Verification items for the finished model (mm, model axes). Give positions to 0.01 mm unless a question says otherwise; leave off trailing zeros. Loops run counter-clockwise (first coordinate to the right, second up) from the corner with the lowest first, then second, coordinate; pieces in that order, holes last. Notation, with made-up numbers: M 47.25,-2.5 L 105.25,-2.5 A20 cw 105.25,26.5 Z; hole C -33,76 d9. An arc over 180 degrees is marked long. Use a Markdown table: item, result.
Solid Edge part; units mm, degrees
sketch "Sketch1" plane through (0, 0, 0) normal (0, 0, 1) x (1, 0, 0)
  line L0 (-35, -25) -> (35, -25)
  line L1 (35, -25) -> (35, 25)
  line L2 (35, 25) -> (-35, 25)
  line L3 (-35, 25) -> (-35, -25)
  dimension "D1" = 35
  dimension "D2" = 35
extrude "Protrusion1" add sketch "Sketch1" along normal blind 20
fillet "Round1" radius 10 4 edges at (-35, -25, 10) (-35, 25, 10) (35, -25, 10) (35, 25, 10)
hole "Hole1" at (-22.5, 0, 20) direction (0, 0, -1) diameter 12 end up to next
hole "Hole2" at (22.5, 0, 20) direction (0, 0, -1) diameter 12 end up to next
properties material "알루미늄, 1060"
(1) Cross-section at C-C on z = 10.5. Record the cut outline in (x, y), then the cut area to 3 significant figures.
Results below:
| item | result |
|---|---|
| outline | M -35,-15 A10 ccw -25,-25 L 25,-25 A10 ccw 35,-15 L 35,15 A10 ccw 25,25 L -25,25 A10 ccw -35,15 Z; hole C -22.5,0 d12; hole C 22.5,0 d12 |
| area | 3,190 mm^2 |
(2) Cross-section at A-A on y = 0. Record the cut outline in (x, z).
Results below:
| item | result |
|---|---|
| outline | M -35,0 L -28.5,0 L -28.5,20 L -35,20 Z; M -16.5,0 L 16.5,0 L 16.5,20 L -16.5,20 Z; M 28.5,0 L 35,0 L 35,20 L 28.5,20 Z |
(3) Material ranges on line 1 (X direction, y = 0, z = 14.75); line 2 (Y direction, x = -22.5, z = 7.5); line 3 (X direction, y = -4, z = 18.25), recorded low to high.
Results below:
| item | result |
|---|---|
| line 1 | -35 to -28.5, -16.5 to 16.5, 28.5 to 35 |
| line 2 | -25 to -6, 6 to 25 |
| line 3 | -35 to -26.97, -18.03 to 18.03, 26.97 to 35 |
(4) Cross-section at D-D on x = 31. Record the cut outline in (y, z).
Results below:
| item | result |
|---|---|
| outline | M -23,0 L 23,0 L 23,20 L -23,20 Z |
(5) Cross-section at B-B on x = 22.5. Record the cut outline in (y, z), then the cut area to 3 significant figures.
Results below:
| item | result |
|---|---|
| outline | M -25,0 L -6,0 L -6,20 L -25,20 Z; M 6,0 L 25,0 L 25,20 L 6,20 Z |
| area | 760 mm^2 |
(6) Draft check along Y on faces 1 (the cylindrical face through (16.643, 1.301, 10.14)), 2 (the flat face through (0, -25, 10)), 3 (the flat face through (0, 25, 10)). Enter one of: +Y half, -Y half, draft (parallel to the pull), parting line (faces both ways), or undercut.
Results below:
| item | result |
|---|---|
| face 1 | undercut |
| face 2 | -Y half |
| face 3 | +Y half |
